```python
from build123d import *

# Parameters (mm, degrees)
F0_W     = 150
F0_H     = 100
F1_DEPTH = 4
F2_W     = 4
F2_H     = 10
F3_DEPTH = 4


with BuildPart() as f1:
    # F0 (on Top) → F1 (new body)
    with BuildSketch(Plane.XY):
        Rectangle(F0_W, F0_H)
    extrude(amount=F1_DEPTH)

    # F2 (on face) → F3 (join)
    with BuildSketch(Plane.XY.offset(4)):
        with Locations((-77, -40)):
            Rectangle(F2_W, F2_H)
        with Locations((-77, -20)):
            Rectangle(F2_W, F2_H)
        with Locations((-77, 0)):
            Rectangle(F2_W, F2_H)
        with Locations((-77, 20)):
            Rectangle(F2_W, F2_H)
        with Locations((-77, 40)):
            Rectangle(F2_W, F2_H)
        with Locations((77, -40)):
            Rectangle(F2_W, F2_H)
        with Locations((77, -20)):
            Rectangle(F2_W, F2_H)
        with Locations((77, 0)):
            Rectangle(F2_W, F2_H)
        with Locations((77, 40)):
            Rectangle(F2_W, F2_H)
        with Locations((77, 20)):
            Rectangle(F2_W, F2_H)
    extrude(amount=-F3_DEPTH)


solid = f1.part
```
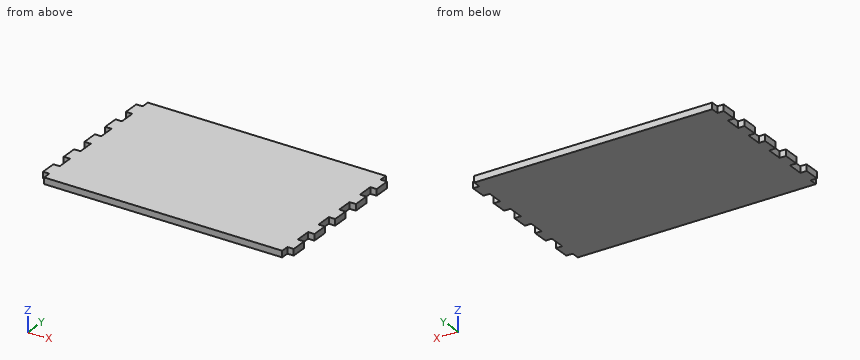
Part model, mm, in its own coordinate system. Round coordinates to 2 decimals unless told otherwise and drop trailing zeros. Order: outer loops, then holes, each group sorted by start corner. A loop starts at its lowest first (then second) coordinate and runs counter-clockwise, first axis right, second up. Notation, with made-up numbers: M 73,89.5 L 93,89.5 A27 ccw 93,121.5 Z; hole C 39.25,-26 d8. An arc over 180 degrees is marked long. Put each result on its own line as item: value. Start each with the question number.
1. Slice it at A-A on y = -7.5. List the corners of the cut face in (x, z).
2. Drill centre line: probe 1 along X at (y, z) = (14.5, 3.35). Where is it in solid material? Low to high. Write a range as [from, to].
3. Drop flat-ended pins along their axis: pin 1 (1.2 mm diameter, centred on x = -76.5, z = 1.5, fed in from +Y); pin 2 (2 mm diameter, centred on y = -46.5, z = 2.5, fed in from -X); pin 3 (2 mm diameter, centred on x = -77.5, z = 1.5, fed in from -Y). Give the stop position or say it passes through.
Findings:
1. outline: M -75,0 L 75,0 L 75,4 L -75,4 Z
2. probe 1: [-75, 75]
3. pin 1: y = 45
3. pin 2: x = -75
3. pin 3: y = -45
